Check sheet for the modelled part. Datum: model origin and axes. Units: mm. Face numbers are marked on the shaded views. A direction names the side the tool comes from. Give positions to 0.01 mm unless a question says otherwise; leave off trailing zeros. Order: outer loops, then holes, each group sorted by start corner. A loop starts at its lowest first (then second) coordinate and runs counter-clockwise, first axis right, second up. Notation, with made-up numbers: M 8,-1 L 34,-1 A29 cw 34,23 Z; hole C 27,-7.5 d4. An arc over 180 degrees is marked long. Answer in a Markdown table with one row per item. Add a question column.
from build123d import *

# Parameters (mm, degrees)
F0_R     = 3.55
F1_DEPTH = 6
F0_R_2   = 2.5
F2_DEPTH = 8


with BuildPart() as f1:
    # F0 (on Top) → F1 (new body)
    with BuildSketch(Plane.XY):
        Polygon((2.5, 4.330127), (-2.5, 4.330127), (-5, 0), (-2.5, -4.330127), (2.5, -4.330127), (5, 0), align=None)
        Circle(F0_R, mode=Mode.SUBTRACT)
    extrude(amount=F1_DEPTH)

    # F0 (on Top) → F2 (join)
    with BuildSketch(Plane.XY):
        Circle(F0_R)
        with Locations((0, 0.79)):
            Circle(F0_R_2, mode=Mode.SUBTRACT)
    extrude(amount=F2_DEPTH)


solid = f1.part
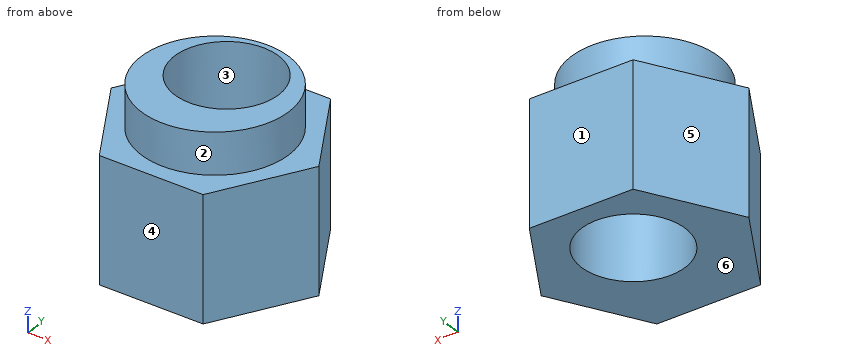
Q1. Tool access check on the marked faces 1 and 2. Record the directions out of +Z, -Z, +X, -X, +Y, -Y that give a thin tool (end or side, any length) a straight path to the whole face; none if there is none.
Q2. Go/stop test with flat-tipped pins: pin 1 (3 mm diameter, centred on y = 2, z = 1, fed in from -X); pin 2 (3 mm diameter, centred on x = 2, y = 0, fed in from -Z); pin 3 (1 mm diameter, centred on y = 2.5, z = 3.5, fed in from +X). Record where each tip stops, or that it passes through.
Q3. Thickness scan on probe 1 along Y at (x, z) = (0, 2.25); probe 2 along X at (y, z) = (-1.5, 1.5); probe 3 along Y at (x, z) = (0.5, 7.5). Record the ranges inside material, lowest first.
Q4. Cross-section at C-C (z = 4.25). Record the boundary of the cut face in (x, y), and give its area (3 significant figures).
Q5. Draft check along Y on the marked faces 3, 4, 5 and 6. Enter one of: pulls with the +Y half, pulls with the -Y half, needs draft (parallel to the pull), parting line crosses it, or undercut.
Q6. Cross-section at D-D (y = -3.25). Record the boundary of the cut face in (x, z).
Q7. Cross-section at B-B (y = 0.5). Record the boundary of the cut face in (x, z), and give its area (3 significant figures).
Q8. Cross-section at A-A (x = 0). Record the boundary of the cut face in (y, z).
Values follow:
| question | item | result |
|---|---|---|
| 1 | face 1 | +Z, -Z, +X, -X, +Y |
| 1 | face 2 | +Z |
| 2 | pin 1 | x = -4.71 |
| 2 | pin 2 | z = 0 |
| 2 | pin 3 | x = 3.85 |
| 3 | probe 1 | -4.33 to -1.71, 3.29 to 4.33 |
| 3 | probe 2 | -4.13 to -1, 1 to 4.13 |
| 3 | probe 3 | -3.51 to -1.66, 3.24 to 3.51 |
| 4 | outline | M -5,0 L -2.5,-4.33 L 2.5,-4.33 L 5,0 L 2.5,4.33 L -2.5,4.33 Z; hole C 0,0.79 d5 |
| 4 | area | 45.3 mm² |
| 5 | face 3 | undercut |
| 5 | face 4 | pulls with the -Y half |
| 5 | face 5 | pulls with the +Y half |
| 5 | face 6 | needs draft |
| 6 | outline | M -3.12,0 L 3.12,0 L 3.12,6 L 1.43,6 L 1.43,8 L -1.43,8 L -1.43,6 L -3.12,6 Z |
| 7 | outline | M -4.71,0 L -2.48,0 L -2.48,8 L -3.51,8 L -3.51,6 L -4.71,6 Z; M 2.48,0 L 4.71,0 L 4.71,6 L 3.51,6 L 3.51,8 L 2.48,8 Z |
| 7 | area | 30.9 mm² |
| 8 | outline | M -4.33,0 L -1.71,0 L -1.71,8 L -3.55,8 L -3.55,6 L -4.33,6 Z; M 3.29,0 L 4.33,0 L 4.33,6 L 3.55,6 L 3.55,8 L 3.29,8 Z |
